```python
from build123d import *

# Parameters (mm, degrees)
F0_R     = 38.1
F0_R_2   = 31.75
F1_DEPTH = 6.35
F3_DEPTH = 33.02
F4_COUNT = 4
F4_ANGLE = 270
F5_R     = 3.175
F6_DEPTH = 25.4


with BuildPart() as f1:
    # F0 (on Right) → F1 (new body)
    with BuildSketch(Plane.YZ):
        Circle(F0_R)
        Circle(F0_R_2, mode=Mode.SUBTRACT)
    extrude(amount=F1_DEPTH)



with BuildPart() as f3:
    # F2 (on Top) → F3 (new body)
    with BuildSketch(Plane.XY):
        Polygon((0, 3.81), (0, 0), (0, -3.81), (6.35, -3.81), (6.35, 3.81), align=None)
    extrude(amount=F3_DEPTH)


with BuildPart() as f1_1:
    add(f1.part)

    add(f3.part)  # F4 merges F3
    # F4: F3 ×4 about axis
    f4_axis = Axis((6.35, 0, 0), (1, 0, 0))
    for i in range(1, F4_COUNT):
        add(f3.part.rotate(f4_axis, i * F4_ANGLE / (F4_COUNT - 1)))

    # F5 (on face) → F6 (cut)
    with BuildSketch(Plane(origin=(0, 0, 0), x_dir=(0, -1, 0), z_dir=(-1, 0, 0))):
        Circle(F5_R)
    extrude(amount=-F6_DEPTH, mode=Mode.SUBTRACT)


solid = f1_1.part
```
Check sheet for the modelled part. Datum: model origin and axes. Units: mm. A direction names the side the tool comes from. Coordinates: 2 decimals unless noted, no trailing zeros. Write each loop counter-clockwise with the first axis right and the second up, starting at its lowest first coordinate (ties: lowest second). Pieces come first, ordered by that corner, then holes. Notation, with made-up numbers: (-31.75, -25.5) -> (18.25, -25.5) arc R6 ccw to (18.25, -18.5) -> close; hole circle Ø5 at (72.5, -36). An arc over 180 degrees is marked (long way). Use a Markdown table: item, result.
1. Sectioned sample at C-C (x = 3.75). Enter the section's corners in (y, z) (3 decimals).
Reported:
| item | result |
|---|---|
| outline | circle Ø76.2 at (0, 0); hole (-31.521, -3.81) arc R31.75 ccw to (-3.81, -31.521) -> (-3.81, -3.81) -> close; hole (-31.521, 3.81) -> (-3.81, 3.81) -> (-3.81, 31.521) arc R31.75 ccw to start; hole circle Ø6.35 at (0, 0); hole (3.81, -31.521) arc R31.75 ccw to (31.521, -3.81) -> (3.81, -3.81) -> close; hole (3.81, 3.81) -> (31.521, 3.81) arc R31.75 ccw to (3.81, 31.521) -> close |
2. Go/stop test with flat-tipped pins: pin 1 Ø3 at (x, z) = (3, -18.5) entering from +Y; pin 2 Ø1 at (x, z) = (2, -27.5) entering from -Y; pin 3 Ø2 at (x, z) = (4.5, 25.5) entering from +Y; pin 4 Ø3 at (y, z) = (8.5, -1) entering from -X. Record where each tip stops, or that it passes through.
Reported:
| item | result |
|---|---|
| pin 1 | stops at y = 34.1 |
| pin 2 | stops at y = -26.88 |
| pin 3 | stops at y = 29.18 |
| pin 4 | stops at x = 0 |
3. Release check for a two-part mould opening along Y. For faces 3 (the flat face through (6.35, -1, -8)), 4 (the flat face through (3, 17, -3.81)), 5 (the cylindrical face through (3.131, -30.235, -23.183)) record: pulls with the +Y half, pulls with the -Y half, needs draft (parallel to the pull), parting line crosses it, or undercut.
Reported:
| item | result |
|---|---|
| face 3 | needs draft |
| face 4 | undercut |
| face 5 | parting line crosses it |
4. Sectioned sample at D-D (y = 23). Enter the section's corners in (x, z), plus the area to 3 significant figures.
Reported:
| item | result |
|---|---|
| outline | (0, -30.37) -> (6.35, -30.37) -> (6.35, -21.89) -> (0, -21.89) -> close; (0, -3.81) -> (6.35, -3.81) -> (6.35, 3.81) -> (0, 3.81) -> close; (0, 21.89) -> (6.35, 21.89) -> (6.35, 30.37) -> (0, 30.37) -> close |
| area | 156 mm2 |
5. Scan lines: line 1 along Z through (x, y) = (4, 0) (3 decimals); line 2 along Z through (x, y) = (4.5, -23); line 3 along Y through (x, z) = (3.25, 4.5). Record each from-to range of solid material in increasing order.
Reported:
| item | result |
|---|---|
| line 1 | z = -38.1 to -3.175, 3.175 to 38.1 |
| line 2 | z = -30.37 to -21.89, -3.81 to 3.81, 21.89 to 30.37 |
| line 3 | y = -37.83 to -31.43, -3.81 to 3.81, 31.43 to 37.83 |
6. Tool access check on faces 1 (the cylindrical face through (3.1, 22.7, 22.2)), 2 (the flat face through (0, 1, 8)). Record the directions out of +Z, -Z, +X, -X, +Y, -Y that give a thin tool (end or side, any length) a straight path to the whole face; none if there is none.
Reported:
| item | result |
|---|---|
| face 1 | +X, -X |
| face 2 | +Z, -Z, -X, +Y, -Y |
7. Sectioned sample at A-A (y = 0). Enter the section's corners in (x, z) (3 decimals), plus the area to 3 significant figures.
Reported:
| item | result |
|---|---|
| outline | (0, -38.1) -> (6.35, -38.1) -> (6.35, -3.175) -> (0, -3.175) -> close; (0, 3.175) -> (6.35, 3.175) -> (6.35, 38.1) -> (0, 38.1) -> close |
| area | 444 mm2 |
